```python
from build123d import *

# Parameters (mm, degrees)
F1_DEPTH = 50
F2_DEPTH = 25
F3_R     = 2


with BuildPart() as f1:
    # F0 (on Front) → F1 (new body)
    with BuildSketch(Plane.XZ):
        with BuildLine():
            Line((-100, -30), (100, -30))
            ThreePointArc((100, -30), (121.2132034356, -21.2132034356), (130, 0))
            ThreePointArc((130, 0), (121.2132034356, 21.2132034356), (100, 30))
            Line((100, 30), (-100, 30))
            ThreePointArc((-100, 30), (-121.2132034356, 21.2132034356), (-130, 0))
            ThreePointArc((-130, 0), (-121.2132034356, -21.2132034356), (-100, -30))
        make_face()
    extrude(amount=F1_DEPTH)

    # F0 (on Front) → F2 (join)
    with BuildSketch(Plane.XZ):
        with BuildLine():
            Line((-100, -50), (100, -50))
            ThreePointArc((100, -50), (135.3553390593, -35.3553390593), (150, 0))
            ThreePointArc((150, 0), (135.3553390593, 35.3553390593), (100, 50))
            Line((100, 50), (-100, 50))
            ThreePointArc((-100, 50), (-135.3553390593, 35.3553390593), (-150, 0))
            ThreePointArc((-150, 0), (-135.3553390593, -35.3553390593), (-100, -50))
        make_face()
        with BuildLine():
            ThreePointArc((130, 0), (121.2132034356, -21.2132034356), (100, -30))
            Line((100, -30), (-100, -30))
            ThreePointArc((-100, -30), (-121.2132034356, -21.2132034356), (-130, 0))
            ThreePointArc((-130, 0), (-121.2132034356, 21.2132034356), (-100, 30))
            Line((-100, 30), (100, 30))
            ThreePointArc((100, 30), (121.2132034356, 21.2132034356), (130, 0))
        make_face(mode=Mode.SUBTRACT)
    extrude(amount=F2_DEPTH)

    # F3
    f3_edges = [f1.edges().sort_by_distance(p)[0] for p in [
        (-150, -25, 0),
        (0, -50, -30),
        (0, -25, -50),
        (150, -25, 0),
        (0, -25, 50),
        (130, -50, 0),
        (0, -50, 30),
        (-130, -50, 0),
    ]]
    fillet(f3_edges, radius=F3_R)


solid = f1.part
```
Input: part model. Units: mm. Frame: model coordinates. A direction names the side the tool comes from. Give positions to 0.01 mm unless a question says otherwise; leave off trailing zeros. Order: outer loops, then holes, each group sorted by start corner. A loop starts at its lowest first (then second) coordinate and runs counter-clockwise, first axis right, second up. Notation, with made-up numbers: M -32.75,26 L 16.25,26 A29 ccw 16.25,65 Z; hole C 72.25,44.5 d9. An arc over 180 degrees is marked long. Return JSON: item names as keys, results as strings.
Item 1: Cut plane A-A (y = -4.5). Return loops of the section in (x, z), then the cut area to 3 significant figures.
Solutions:
{"outline": "M -100,-50 L 100,-50 A50 ccw 100,50 L -100,50 A50 ccw Z", "area": "27,900 mm^2"}
Item 2: Access query for faces 1 (the cylindrical face through (-129.993, -36.339, 0.66)), 2 (the flat face through (-1, -36, -30)), 3 (the cylindrical face through (129.993, -36.339, -0.66)). Directions: +Z, -Z, +X, -X, +Y, -Y. A direction counts if a zero-diameter tool reaches every point of the face in a straight line with its end or side. Return the directions, or none.
Solutions:
{"face 1": "-X, -Y", "face 2": "-Z, +X, -X, -Y", "face 3": "+X, -Y"}
Item 3: First-contact query: P1, Ø5, axis at x = 57, z = 35, coming from the -Y side; P2, Ø7, axis at x = -42.5, y = -42, coming from the -Z side; P3, Ø7, axis at x = 10, y = -32.5, coming from the +Z side. Flat tips, straight axial feed; report the tip coordinate or a pass-through.
Solutions:
{"P1": "y = -25", "P2": "z = -30", "P3": "z = 30"}
Item 4: Cut plane B-B (y = -36). Return loops of the section in (x, z), then the cut area to 3 significant figures.
Solutions:
{"outline": "M -100,-30 L 100,-30 A30 ccw 100,30 L -100,30 A30 ccw Z", "area": "14,800 mm^2"}
Item 5: Ray query, probe 1 along Y at (x, z) = (14.5, -39); probe 2 along Z at (x, y) = (-49.5, -33.5); probe 3 along Z at (x, y) = (-114, -41). Return the intervals inside material, ascending.
Solutions:
{"probe 1": "-25 to 0", "probe 2": "-30 to 30", "probe 3": "-26.53 to 26.53"}
